from build123d import *

# Parameters (mm, degrees)
F1_DEPTH    = 25
F2_R        = 1.6
F3_DEPTH    = 2
F4_F1_R     = 3
F4_T2_DEPTH = 17
F4_T4_DEPTH = 26.2
F4_T6_DEPTH = 40


# Not quite as in the source:
# - a fillet or chamfer that OpenCascade refuses, or shapes differently, is made with other operations: its cross-section is extruded or revolved along the edge and cut away or added


with BuildPart() as f1:
    # F0 (on Front) → F1 (new body)
    with BuildSketch(Plane.XZ):
        Polygon((0, 2), (0, 0), (7, 0), (7, 11.2), (3, 11.2), (3, 9.2), (4.5, 9.2), (4.5, 5.6), (5, 5.6), (5, 2), align=None)
    extrude(amount=F1_DEPTH)

    # F2 (on Top) → F3 (join)
    with BuildSketch(Plane.XY):
        with BuildLine():
            Line((15, -9.5), (8.5, -9.5))
            ThreePointArc((8.5, -9.5), (7.4393398282, -9.0606601718), (7, -8))
            Line((7, -8), (0, -8))
            Line((0, -8), (0, -9.5))
            Line((0, -9.5), (0, -15.5))
            Line((0, -15.5), (0, -17))
            Line((0, -17), (7, -17))
            ThreePointArc((7, -17), (7.4393398282, -15.9393398282), (8.5, -15.5))
            Line((8.5, -15.5), (15, -15.5))
            Line((15, -15.5), (15, -9.5))
        make_face()
        with Locations((12, -12.5)):
            Circle(F2_R, mode=Mode.SUBTRACT)
    extrude(amount=F3_DEPTH)

    # F4: fillet of radius 3 on 6 edges, made by hand

    # F4_f1
    f4_f1_edges = [f1.edges().sort_by_distance(p)[0] for p in [
        (7, -12.5, 2),
    ]]
    fillet(f4_f1_edges, radius=F4_F1_R)

    # F4_s3 → F4_t2 (cut)
    with BuildSketch(Plane.XY.offset(-7.5)):
        with BuildLine():
            ThreePointArc((15, -12.5), (14.1213203436, -14.6213203436), (12, -15.5))
            Line((12, -15.5), (12, -15.56))
            Line((12, -15.56), (15.06, -15.56))
            Line((15.06, -15.56), (15.06, -12.5))
            Line((15.06, -12.5), (15, -12.5))
        make_face()
        with BuildLine():
            ThreePointArc((12, -9.5), (14.1213203436, -10.3786796564), (15, -12.5))
            Line((15, -12.5), (15.06, -12.5))
            Line((15.06, -12.5), (15.06, -9.44))
            Line((15.06, -9.44), (12, -9.44))
            Line((12, -9.44), (12, -9.5))
        make_face()
    extrude(amount=F4_T2_DEPTH, mode=Mode.SUBTRACT)

    # F4_s5 → F4_t4 (cut)
    with BuildSketch(Plane.XY.offset(-7.5)):
        with BuildLine():
            ThreePointArc((7, -22), (6.1213203436, -24.1213203436), (4, -25))
            Line((4, -25), (4, -25.06))
            Line((4, -25.06), (7.06, -25.06))
            Line((7.06, -25.06), (7.06, -22))
            Line((7.06, -22), (7, -22))
        make_face()
        with BuildLine():
            ThreePointArc((7, -3), (6.1213203436, -0.8786796564), (4, 0))
            Line((4, 0), (4, 0.06))
            Line((4, 0.06), (7.06, 0.06))
            Line((7.06, 0.06), (7.06, -3))
            Line((7.06, -3), (7, -3))
        make_face()
    extrude(amount=F4_T4_DEPTH, mode=Mode.SUBTRACT)

    # F4_s7 → F4_t6 (cut)
    with BuildSketch(Plane.XZ.offset(-7.5)):
        with BuildLine():
            ThreePointArc((7, 8.2), (6.1213203436, 10.3213203436), (4, 11.2))
            Line((4, 11.2), (4, 11.26))
            Line((4, 11.26), (7.06, 11.26))
            Line((7.06, 11.26), (7.06, 8.2))
            Line((7.06, 8.2), (7, 8.2))
        make_face()
    extrude(amount=F4_T6_DEPTH, mode=Mode.SUBTRACT)

    # F5: F1 across face


with BuildPart() as f1_1:
    add(f1.part)
    add(f1.part.mirror(Plane(origin=(0, -12.5, 1), x_dir=(0, -1, 0), z_dir=(-1, 0, 0))))


solid = f1_1.part
Geometry check sheet. Reference: the model listing, model coordinates, mm. A direction names the side the tool comes from. Round coordinates to 2 decimals unless told otherwise and drop trailing zeros. Write each loop counter-clockwise with the first axis right and the second up, starting at its lowest first coordinate (ties: lowest second). Pieces come first, ordered by that corner, then holes.
Item 1: Section check A-A (z = 1.5). Record the boundary of the cut face in (x, y), plus the area to 3 significant figures.
Determined:
outline: (-12, -15.5) - (-8.5, -15.5) arc R1.5 cw to (-7, -17) - (-7, -22) arc R3 ccw to (-4, -25) - (4, -25) arc R3 ccw to (7, -22) - (7, -17) arc R1.5 cw to (8.5, -15.5) - (12, -15.5) arc R3 ccw to (12, -9.5) - (8.5, -9.5) arc R1.5 cw to (7, -8) - (7, -3) arc R3 ccw to (4, 0) - (-4, 0) arc R3 ccw to (-7, -3) - (-7, -8) arc R1.5 cw to (-8.5, -9.5) - (-12, -9.5) arc R3 ccw to start; hole circle Ø3.2 at (-12, -12.5); hole circle Ø3.2 at (12, -12.5)
area: 416 mm2
Item 2: Section check D-D (x = -12.5). Record the boundary of the cut face in (y, z).
Determined:
outline: (-15.46, 0) - (-14.02, 0) - (-14.02, 2) - (-15.46, 2) - close; (-10.98, 0) - (-9.54, 0) - (-9.54, 2) - (-10.98, 2) - close
Item 3: Go/stop test with flat-tipped pins: pin 1 Ø4 at (x, y) = (12.5, -13.5) entering from +Z; pin 2 Ø1 at (y, z) = (-9, 10) entering from +X; pin 3 Ø3 at (y, z) = (-13.5, 9) entering from +X. Record where each tip stops, or that it passes through.
Determined:
pin 1: stops at z = 2
pin 2: stops at x = 6.7
pin 3: stops at x = 7
Item 4: Section check C-C (y = -7.25). Record the boundary of the cut face in (x, z), plus the area to 3 significant figures.
Determined:
outline: (-7, 0) - (7, 0) - (7, 8.2) arc R3 ccw to (4, 11.2) - (3, 11.2) - (3, 9.2) - (4.5, 9.2) - (4.5, 5.6) - (5, 5.6) - (5, 2) - (-5, 2) - (-5, 5.6) - (-4.5, 5.6) - (-4.5, 9.2) - (-3, 9.2) - (-3, 11.2) - (-4, 11.2) arc R3 ccw to (-7, 8.2) - close
area: 72.5 mm2
Item 5: Section check B-B (z = 10). Record the boundary of the cut face in (x, y).
Determined:
outline: (-6.4, -23.8) arc R3 ccw to (-4, -25) - (-3, -25) - (-3, 0) - (-4, 0) arc R3 ccw to (-6.4, -1.2) - close; (3, -25) - (4, -25) arc R3 ccw to (6.4, -23.8) - (6.4, -1.2) arc R3 ccw to (4, 0) - (3, 0) - close
Item 6: Access from +Z, -Z, +X, -X, +Y, -Y to the whole of each face (thin tool, end or side, straight path). Record for faces 1 (the face through (-10, -9.5, 1)), 2 (the face through (-7, -12, 6)), 3 (the face through (10, -15.5, 1)), 4 (the face through (10, -9.5, 1)), 5 (the face through (14, -13, 2)).
Determined:
face 1: +Z, -Z, -X, +Y
face 2: +Z, -X
face 3: +Z, -Z, +X, -Y
face 4: +Z, -Z, +X, +Y
face 5: +Z, +X, +Y, -Y
Item 7: Mould release check, pull along X, two halves, no side actions. Record for faces 6 (the face through (5, -12, 4)), 7 (the face through (6.14, -12.32, 10.3)), 8 (the face through (-3, -12, 10)), 9 (the face through (-3.5, -12.3, 11.2)): +X half, -X half, draft (parallel to the pull), parting line (faces both ways), or undercut.
Determined:
face 6: undercut
face 7: +X half
face 8: undercut
face 9: draft
Item 8: Material ranges on line 1 along Y through (x, z) = (12, 1.2); line 2 along Z through (x, y) = (3.75, -7.25); line 3 along X through (y, z) = (-5.75, 3.5), recorded low to high.
Determined:
line 1: y = -15.5 to -14.1, -10.9 to -9.5
line 2: z = 0 to 2, 9.2 to 11.2
line 3: x = -7 to -5, 5 to 7
